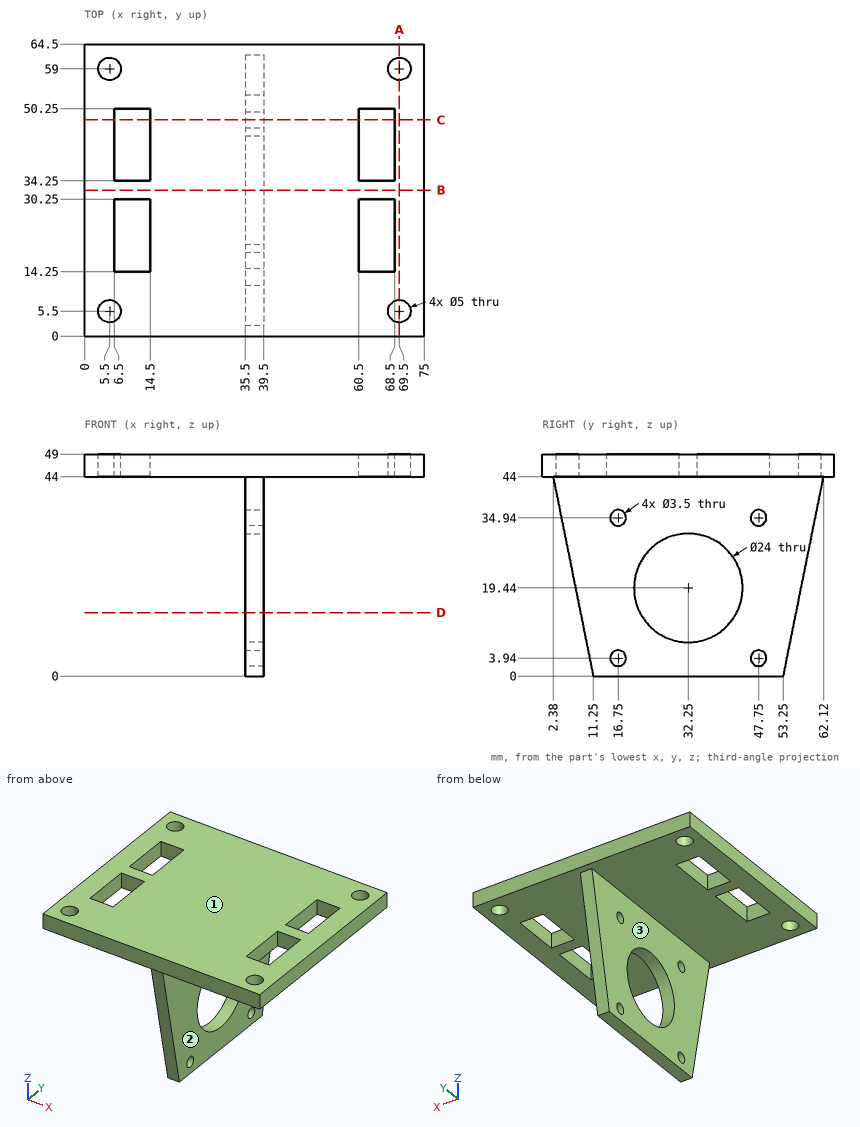
Check sheet for the drawn part. Datum: minimum x, y, z corner. Units: mm. A direction names the side the tool comes from. Round coordinates to 2 decimals unless told otherwise and drop trailing zeros. Write each loop counter-clockwise with the first axis right and the second up, starting at its lowest first coordinate (ties: lowest second). Pieces come first, ordered by that corner, then holes. Notation, with made-up numbers: (36, 86) -> (65, 86) arc R26 ccw to (65, 106) -> close; hole circle Ø6 at (55, -4.5). An arc over 180 degrees is marked (long way). One line per item, written item: value. Start each with the question number.
(1) Go/stop test with flat-tipped pins: pin 1 Ø8 at (x, y) = (69.5, 5.5) entering from -Z; pin 2 Ø8 at (y, z) = (9.5, 21) entering from +X; pin 3 Ø4 at (y, z) = (16.75, 34.94) entering from -X. Record where each tip stops, or that it passes through.
(2) Cross-section at A-A, the plane x = 69.5. Record the cut outline in (y, z).
(3) Cross-section at D-D, the plane z = 14. Record the cut outline in (x, y), and give its area (3 significant figures).
(4) Access from +Z, -Z, +X, -X, +Y, -Y to the whole of each face (thin tool, end or side, straight path). Record for the marked faces 1, 2 and 3.
(5) Cross-section at C-C, the plane y = 47.75. Record the cut outline in (x, z).
(6) Scan lines: line 1 (Y direction, x = 5.5, z = 46.6); line 2 (Z direction, x = 36, y = 32); line 3 (X direction, y = 14.5, z = 6.5). Record each from-to range of solid material in increasing order. Write a range as [from, to].
(7) Cross-section at B-B, the plane y = 32.25. Record the cut outline in (x, z).
Answer:
1. pin 1: z = 44
1. pin 2: x = 39.5
1. pin 3: x = 35.5
2. outline: (0, 44) -> (3, 44) -> (3, 49) -> (0, 49) -> close; (8, 44) -> (56.5, 44) -> (56.5, 49) -> (8, 49) -> close; (61.5, 44) -> (64.5, 44) -> (64.5, 49) -> (61.5, 49) -> close
3. outline: (35.5, 8.43) -> (39.5, 8.43) -> (39.5, 21.55) -> (35.5, 21.55) -> close; (35.5, 42.95) -> (39.5, 42.95) -> (39.5, 56.07) -> (35.5, 56.07) -> close
3. area: 105 mm²
4. face 1: +Z, +X, -X, +Y, -Y
4. face 2: -Z, +X, +Y, -Y
4. face 3: -Z, -X, +Y, -Y
5. outline: (0, 44) -> (6.5, 44) -> (6.5, 49) -> (0, 49) -> close; (14.5, 44) -> (35.5, 44) -> (35.5, 36.69) -> (39.5, 36.69) -> (39.5, 44) -> (60.5, 44) -> (60.5, 49) -> (14.5, 49) -> close; (35.5, 0) -> (39.5, 0) -> (39.5, 2.19) -> (35.5, 2.19) -> close; (35.5, 5.69) -> (39.5, 5.69) -> (39.5, 33.19) -> (35.5, 33.19) -> close; (68.5, 44) -> (75, 44) -> (75, 49) -> (68.5, 49) -> close
6. line 1: [0, 3], [8, 56.5], [61.5, 64.5]
6. line 2: [0, 7.44], [31.44, 49]
6. line 3: [35.5, 39.5]
7. outline: (0, 44) -> (35.5, 44) -> (35.5, 31.44) -> (39.5, 31.44) -> (39.5, 44) -> (75, 44) -> (75, 49) -> (0, 49) -> close; (35.5, 0) -> (39.5, 0) -> (39.5, 7.44) -> (35.5, 7.44) -> close
